Part model, mm, in its own coordinate system. A direction names the side the tool comes from. Coordinates: 2 decimals unless noted, no trailing zeros. Write each loop counter-clockwise with the first axis right and the second up, starting at its lowest first coordinate (ties: lowest second). Pieces come first, ordered by that corner, then holes. Notation, with made-up numbers: (29.5, -12.5) - (44.5, -12.5) arc R32 ccw to (44.5, 25.5) - close; hole circle Ø1 at (-37, 24). An arc over 180 degrees is marked (long way). Use a Markdown table: item, result.
```python
from build123d import *

# Parameters (mm, degrees)
F0_W     = 24
F0_H     = 24
F1_DEPTH = 2
F2_DEPTH = 10
F3_SIZE2 = 9.99999
F3_SIZE  = 5.49999
F4_SIZE2 = 9.99999
F4_SIZE  = 5.49999
F5_W     = 8
F5_H     = 2
F6_DEPTH = 25


# Not quite as in the source:
# - a fillet or chamfer is up to 0.001 mm smaller than in the source, because OpenCascade refuses the exact size


with BuildPart() as f1:
    # F0 (on Top) → F1 (new body)
    with BuildSketch(Plane.XY):
        Rectangle(F0_W, F0_H)
        Polygon((-6, -10), (-6, -2.5), (-4, -2.5), (-4, -8), (0, -8), (4, -8), (4, -2.5), (6, -2.5), (6, -10), (0, -10), align=None, mode=Mode.SUBTRACT)
        Polygon((-4, 2.5), (-6, 2.5), (-6, 10), (0, 10), (6, 10), (6, 2.5), (4, 2.5), (4, 8), (0, 8), (-4, 8), align=None, mode=Mode.SUBTRACT)
        Polygon((-6, 10), (-6, 2.5), (-4, 2.5), (-4, 8), (0, 8), (4, 8), (4, 2.5), (6, 2.5), (6, 10), (0, 10), align=None)
        Polygon((-4, -2.5), (-6, -2.5), (-6, -10), (0, -10), (6, -10), (6, -2.5), (4, -2.5), (4, -8), (0, -8), (-4, -8), align=None)
    extrude(amount=-F1_DEPTH)

    # F0 (on Top) → F2 (join)
    with BuildSketch(Plane.XY):
        Polygon((-6, 10), (-6, 2.5), (-4, 2.5), (-4, 8), (0, 8), (4, 8), (4, 2.5), (6, 2.5), (6, 10), (0, 10), align=None)
        Polygon((-4, -2.5), (-6, -2.5), (-6, -10), (0, -10), (6, -10), (6, -2.5), (4, -2.5), (4, -8), (0, -8), (-4, -8), align=None)
    extrude(amount=F2_DEPTH)

    # F3 (size 5.5 and 10 in the source; OpenCascade refuses exactly that, so slightly less here)
    f3_edges = [f1.edges().sort_by_distance(p)[0] for p in [
        (-5, 2.5, 10),
        (5, 2.5, 10),
    ]]
    f3_side = f1.faces().sort_by_distance((-5.85849, 6.25, 10))[0]
    chamfer(f3_edges, length=F3_SIZE, length2=F3_SIZE2, reference=f3_side)

    # F4 (size 5.5 and 10 in the source; OpenCascade refuses exactly that, so slightly less here)
    f4_edges = [f1.edges().sort_by_distance(p)[0] for p in [
        (5, -2.5, 10),
        (-5, -2.5, 10),
    ]]
    f4_side = f1.faces().sort_by_distance((-5, -2.64151, 10))[0]
    chamfer(f4_edges, length=F4_SIZE, length2=F4_SIZE2, reference=f4_side)

    # F5 (on face) → F6 (cut)
    with BuildSketch(Plane.XZ.offset(10)):
        with Locations((0, 7)):
            Rectangle(F5_W, F5_H)
    extrude(amount=-F6_DEPTH, mode=Mode.SUBTRACT)


solid = f1.part
```
Item 1: Band-saw the part on B-B, the plane y = -9.5. Give the cut face in (x, z), then the cut area to 3 significant figures.
From the geometry:
| item | result |
|---|---|
| outline | (-12, -2) - (12, -2) - (12, 0) - (6, 0) - (6, 10) - (-6, 10) - (-6, 0) - (-12, 0) - close; hole (-4, 6) - (4, 6) - (4, 8) - (-4, 8) - close |
| area | 152 mm^2 |
Item 2: Two-plate mould, pull along X, no slides. Class faces 1 (the face through (0, -8, 9)), 2 (the face through (0, 0, -2)), 3 (the face through (-6, 7, 4)), 4 (the face through (0, 8, 3)): pulls with the +X half, pulls with the -X half, needs draft (parallel to the pull), parting line crosses it, or undercut.
From the geometry:
| item | result |
|---|---|
| face 1 | undercut |
| face 2 | needs draft |
| face 3 | pulls with the -X half |
| face 4 | undercut |
Item 3: Which spindle directions (+Z, -Z, +X, -X, +Y, -Y) get a long thin tool onto all of the face, cutting with end or side? Do faces 5 (the face through (0, -10, 5)), 6 (the face through (0, -9, 8)), 7 (the face through (5.01, -5.21, 4.93)). Say none if no direction does.
From the geometry:
| item | result |
|---|---|
| face 5 | +Z, +X, -X, -Y |
| face 6 | +Y, -Y |
| face 7 | +Z, +X, -X |
Item 4: Band-saw the part on A-A, the plane z = 2. Give the cut face in (x, y).
From the geometry:
| item | result |
|---|---|
| outline | (-6, -10) - (6, -10) - (6, -3.6) - (4, -3.6) - (4, -8) - (-4, -8) - (-4, -3.6) - (-6, -3.6) - close; (-6, 3.6) - (-4, 3.6) - (-4, 8) - (4, 8) - (4, 3.6) - (6, 3.6) - (6, 10) - (-6, 10) - close |
Item 5: Band-saw the part on C-C, the plane x = 1.5. Give the cut face in (y, z), then the cut area to 3 significant figures.
From the geometry:
| item | result |
|---|---|
| outline | (-12, -2) - (12, -2) - (12, 0) - (10, 0) - (10, 6) - (8, 6) - (8, 0) - (-8, 0) - (-8, 6) - (-10, 6) - (-10, 0) - (-12, 0) - close; (-10, 8) - (-8, 8) - (-8, 10) - (-10, 10) - close; (8, 8) - (10, 8) - (10, 10) - (8, 10) - close |
| area | 80.0 mm^2 |
Item 6: Drill centre lines: probe 1 along Y at (x, z) = (0.75, 2.5); probe 2 along Z at (x, y) = (0, 9); probe 3 along X at (y, z) = (-7, 2.75). Where is each one in solid material? Low to high.
From the geometry:
| item | result |
|---|---|
| probe 1 | -10 to -8, 8 to 10 |
| probe 2 | -2 to 6, 8 to 10 |
| probe 3 | -6 to -4, 4 to 6 |
Item 7: Drop flat-ended pins along their axis: P1, Ø6, axis at y = -6, z = 7.5, coming from the +X side; P2, Ø2, axis at y = -7.5, z = 6, coming from the -X side; P3, Ø6, axis at x = -5, z = 8.5, coming from the +Y side. Give the stop position or say it passes through.
From the geometry:
| item | result |
|---|---|
| P1 | x = 6 |
| P2 | x = -6 |
| P3 | y = 10 |
